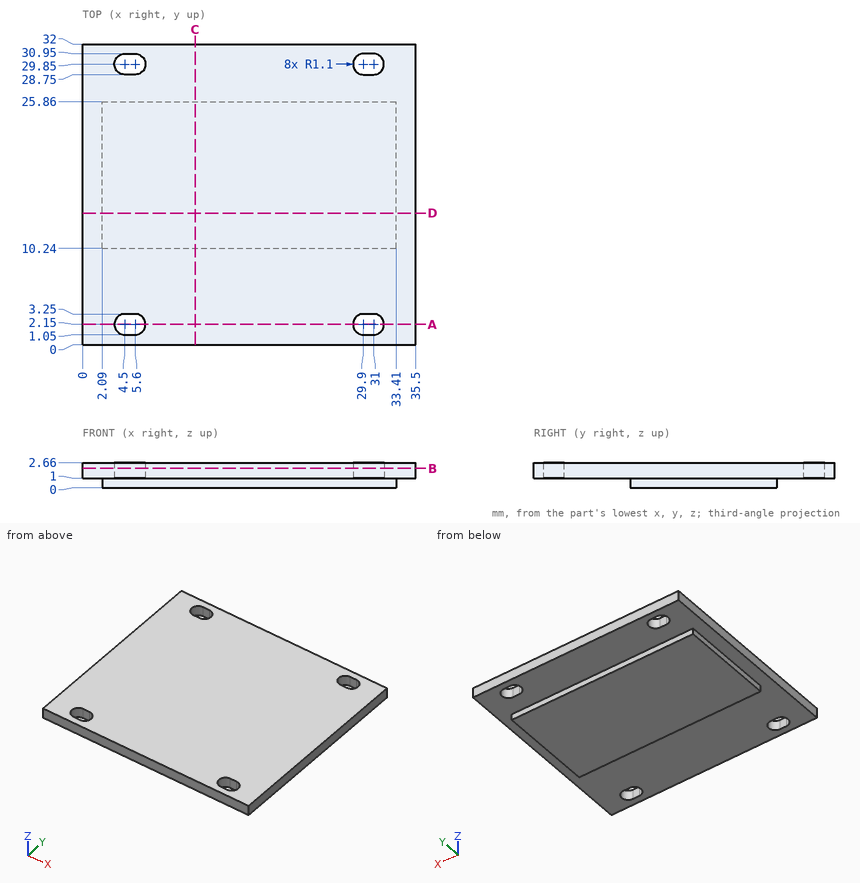
Could you check a few things on this drawing? It's one solid part, dimensions in mm from its lowest x, y, z. Give positions to 0.01 mm unless a question says otherwise; leave off trailing zeros. Write each loop counter-clockwise with the first axis right and the second up, starting at its lowest first coordinate (ties: lowest second). Pieces come first, ordered by that corner, then holes. Notation, with made-up numbers: (-37.5, 12.5) -> (-28.5, 12.5) arc R22 ccw to (-28.5, 44.5) -> close; hole circle Ø1 at (-24.75, 66). An arc over 180 degrees is marked (long way). Answer as a JSON object with one key per item and string values.
Q1. Suppose I cut it at C-C on x = 12. Write out the boundary of the cut face in (y, z).
Taken from the geometry:
{"outline": "(0, 1) -> (10.24, 1) -> (10.24, 0) -> (25.86, 0) -> (25.86, 1) -> (32, 1) -> (32, 2.66) -> (0, 2.66) -> close"}
Q2. Please list where these lines run through material, in increasing order: L1, parallel to Y at x = 30, z = 1.6; L2, parallel to Y at x = 9.5, z = 0.3.
Taken from the geometry:
{"L1": "y = 0 to 1.05, 3.25 to 28.75, 30.95 to 32", "L2": "y = 10.24 to 25.86"}
Q3. Suppose I cut it at D-D on y = 14. Write out the boundary of the cut face in (x, z).
Taken from the geometry:
{"outline": "(0, 1) -> (2.09, 1) -> (2.09, 0) -> (33.41, 0) -> (33.41, 1) -> (35.5, 1) -> (35.5, 2.66) -> (0, 2.66) -> close"}
Q4. Will these pins go through, and if not, where does the flat tip stop? pin 1 Ø0.8 at (x, z) = (12.5, 0.5) entering from +Y; pin 2 Ø0.8 at (y, z) = (21.5, 0.5) entering from -X.
Taken from the geometry:
{"pin 1": "stops at y = 25.86", "pin 2": "stops at x = 2.09"}
Q5. Suppose I cut it at B-B on z = 2.05. Write out the boundary of the cut face in (x, y), then the cut area to 3 significant figures.
Taken from the geometry:
{"outline": "(0, 0) -> (35.5, 0) -> (35.5, 32) -> (0, 32) -> close; hole (4.5, 1.05) -> (5.6, 1.05) arc R1.1 ccw to (5.6, 3.25) -> (4.5, 3.25) arc R1.1 ccw to start; hole (4.5, 28.75) -> (5.6, 28.75) arc R1.1 ccw to (5.6, 30.95) -> (4.5, 30.95) arc R1.1 ccw to start; hole (29.9, 1.05) -> (31, 1.05) arc R1.1 ccw to (31, 3.25) -> (29.9, 3.25) arc R1.1 ccw to start; hole (29.9, 28.75) -> (31, 28.75) arc R1.1 ccw to (31, 30.95) -> (29.9, 30.95) arc R1.1 ccw to start", "area": "1,110 mm²"}
Q6. Suppose I cut it at A-A on y = 2.15. Write out the boundary of the cut face in (x, z).
Taken from the geometry:
{"outline": "(0, 1) -> (3.4, 1) -> (3.4, 2.66) -> (0, 2.66) -> close; (6.7, 1) -> (28.8, 1) -> (28.8, 2.66) -> (6.7, 2.66) -> close; (32.1, 1) -> (35.5, 1) -> (35.5, 2.66) -> (32.1, 2.66) -> close"}
